from build123d import *

# Parameters (mm, degrees)
SKETCH1_W                = 21.5
SKETCH1_H                = 21.5
SKETCH1_W_2              = 20
SKETCH1_H_2              = 20
BOSS_EXTRUDE1_DEPTH      = 7
SKETCH1_3_W              = 20
SKETCH1_3_H              = 9.25
SKETCH1_3_H_2            = 1.5
BOSS_EXTRUDE2_DEPTH      = 0.75
SKETCH1_4_W              = 20
SKETCH1_4_H              = 1.5
BOSS_EXTRUDE3_DEPTH      = 12
BOSS_EXTRUDE4_DEPTH      = 5
BOSS_EXTRUDE4_DEPTH_BACK = 6.5
SKETCH3_W                = 20
SKETCH3_H                = 2
CUT_EXTRUDE1_DEPTH       = 11


with BuildPart() as part:
    # Sketch1 → Boss-Extrude1 (new body)
    with BuildSketch(Plane(origin=(0, 0, 0), x_dir=(1, 0, 0), z_dir=(0, 1, 0))):
        Rectangle(SKETCH1_W, SKETCH1_H)
        Rectangle(SKETCH1_W_2, SKETCH1_H_2, mode=Mode.SUBTRACT)
    extrude(amount=BOSS_EXTRUDE1_DEPTH)

    # Sketch1_3 → Boss-Extrude2 (add)
    with BuildSketch(Plane(origin=(0, 0, 0), x_dir=(1, 0, 0), z_dir=(0, 1, 0))):
        with Locations((0, -5.375)):
            Rectangle(SKETCH1_3_W, SKETCH1_3_H)
        Rectangle(SKETCH1_3_W, SKETCH1_3_H_2)
        with Locations((0, 5.375)):
            Rectangle(SKETCH1_3_W, SKETCH1_3_H)
    extrude(amount=BOSS_EXTRUDE2_DEPTH)

    # Sketch1_4 → Boss-Extrude3 (add)
    with BuildSketch(Plane(origin=(0, 0, 0), x_dir=(1, 0, 0), z_dir=(0, 1, 0))):
        Rectangle(SKETCH1_4_W, SKETCH1_4_H)
    extrude(amount=BOSS_EXTRUDE3_DEPTH)

    # Sketch3 → Boss-Extrude4 (add, two sides: drawn at the far end of the back side and taken through both)
    with BuildSketch(Plane(origin=(0, 0, -0.75), x_dir=(-1, 0, 0), z_dir=(0, 0, -1)).offset(-BOSS_EXTRUDE4_DEPTH_BACK)):
        with Locations((0, 11)):
            Rectangle(SKETCH3_W, SKETCH3_H)
    extrude(amount=BOSS_EXTRUDE4_DEPTH + BOSS_EXTRUDE4_DEPTH_BACK)

    # Sketch4 → Cut-Extrude1 (cut)
    with BuildSketch(Plane(origin=(0, 12, 0), x_dir=(1, 0, 0), z_dir=(0, 1, 0))):
        Polygon((-8.507158245, 3.482615691), (8.492841755, 3.517384309), (8.507158245, -3.482615691), (-8.492841755, -3.517384309), align=None)
    extrude(amount=-CUT_EXTRUDE1_DEPTH, mode=Mode.SUBTRACT)


solid = part.part
CAD build for the part. Positions are in the model's coordinates, mm. A direction names the side the tool comes from. Coordinates: 2 decimals unless noted, no trailing zeros. Order: outer loops, then holes, each group sorted by start corner. A loop starts at its lowest first (then second) coordinate and runs counter-clockwise, first axis right, second up.
Item 1: Pin check, flat tips, straight feed: pin 1 Ø2.5 at (y, z) = (10.5, 1.5) entering from +X; pin 2 Ø1 at (x, y) = (0, 11.5) entering from +Z; pin 3 Ø1.5 at (y, z) = (10.5, 1) entering from -X. Stop position of each tip, or through.
Check sheet entries:
pin 1: stops at x = 10
pin 2: stops at z = 5.75
pin 3: stops at x = -10
Item 2: Band-saw the part on B-B on z = -8.25. List the corners of the cut face in (x, y), plus the area to 3 significant figures.
Check sheet entries:
outline: (-10.75, 0) - (10.75, 0) - (10.75, 7) - (10, 7) - (10, 0.75) - (-10, 0.75) - (-10, 7) - (-10.75, 7) - close
area: 25.5 mm2
Item 3: Band-saw the part on D-D on y = 7.75. List the corners of the cut face in (x, z).
Check sheet entries:
outline: (-10, -0.75) - (-8.5, -0.75) - (-8.5, 0.75) - (-10, 0.75) - close; (8.5, -0.75) - (10, -0.75) - (10, 0.75) - (8.5, 0.75) - close
Item 4: Two-plate mould, pull along Y, no slides. Class faces 6 (the face through (0, 10, 4)), 7 (the face through (-0.8, 7, 10.3)), 8 (the face through (0, 11, -5.75)): +Y half, -Y half, draft (parallel to the pull), parting line (faces both ways), or undercut.
Check sheet entries:
face 6: undercut
face 7: +Y half
face 8: draft
Item 5: Drill centre lines: L1, parallel to Y at x = -8.25, z = 4.25; L2, parallel to Z at x = 2.5, y = 4. Where is each one in solid material? Low to high.
Check sheet entries:
L1: y = 0 to 0.75, 10 to 12
L2: z = -10.75 to -10, 10 to 10.75
Item 6: Band-saw the part on A-A on z = -4.5. List the corners of the cut face in (x, y).
Check sheet entries:
outline: (-10.75, 0) - (10.75, 0) - (10.75, 7) - (10, 7) - (10, 0.75) - (-10, 0.75) - (-10, 7) - (-10.75, 7) - close; (-10, 10) - (10, 10) - (10, 12) - (-10, 12) - close
Item 7: 3-axis set-ups, long thin cutter, end or side, ignore diameter. For faces 1 (the face through (0, 4, -10)), 2 (the face through (-10, 11, 0)), 3 (the face through (10, 11, 0)), 4 (the face through (10, 4, 5)), 5 (the face through (10.75, 3, 0)): which of +Z, -Z, +X, -X, +Y, -Y reach the whole face in a straight line?
Check sheet entries:
face 1: +Y
face 2: +Z, -Z, -X, +Y
face 3: +Z, -Z, +X, +Y
face 4: none
face 5: +Z, -Z, +X, +Y, -Y
Item 8: Band-saw the part on C-C on x = -0.5. List the corners of the cut face in (y, z).
Check sheet entries:
outline: (0, -10.75) - (7, -10.75) - (7, -10) - (0.75, -10) - (0.75, -0.75) - (1, -0.75) - (1, 0.75) - (0.75, 0.75) - (0.75, 10) - (7, 10) - (7, 10.75) - (0, 10.75) - close; (10, -5.75) - (12, -5.75) - (12, -3.5) - (10, -3.5) - close; (10, 3.5) - (12, 3.5) - (12, 5.75) - (10, 5.75) - close
